Geometry check sheet. Reference: the model listing, model coordinates, mm. A direction names the side the tool comes from. Round coordinates to 2 decimals unless told otherwise and drop trailing zeros. Loops run counter-clockwise (first coordinate to the right, second up) from the corner with the lowest first, then second, coordinate; pieces in that order, holes last. Notation, with made-up numbers: (52.5, 42) - (80.5, 42) arc R31 cw to (80.5, 75) - close; hole circle Ø6 at (40.5, 63). An arc over 180 degrees is marked (long way). Answer as CSV lines item,"result". Start each with the question number.
1) Cross-section at B-B on x = 0. Record the boundary of the cut face in (y, z).
2) Depth check by flat-ended pin: P1, Ø1, axis at x = 1.5, z = 2.5, coming from the +Y side; P2, Ø4, axis at x = 4, y = 6.5, coming from the +Z side; P3, Ø3.5, axis at x = 0, z = 0, coming from the +Y side; P4, Ø2, axis at y = 20, z = 1.5, coming from the +X side. Enter the tip coordinate at first touch or a pass-through.
3) Cross-section at A-A on z = 0. Record the boundary of the cut face in (x, y).
4) Cross-section at C-C on y = 7. Record the boundary of the cut face in (x, z).
5) Draft check along Z on faces 3 (the flat face through (-2.1, 0, 4.3)), 4 (the cylindrical face through (0.9, 17.6, 2.86)), 5 (the cylindrical face through (-9.76, 12.32, -2.17)). Enter one of: released by +Z, released by -Z, zero draft, split by the parting line, or undercut.
6) Cross-section at D-D on y = 15.5. Record the boundary of the cut face in (x, z), and give its area (3 significant figures).
7) Thickness scan on line 1 along X through (y, z) = (7.25, 0); line 2 along X through (y, z) = (14, 0); line 3 along Y through (x, z) = (-4, 2). Record the ranges inside material, lowest first.
8) Access from +Z, -Z, +X, -X, +Y, -Y to the whole of each face (thin tool, end or side, straight path). Record for faces 1 (the flat face through (2.4, 25, 2.1)), 2 (the cylindrical face through (1.352, 4.93, -4.292)).
from build123d import *

# Parameters (mm, degrees)
SKETCH1_R           = 10
BOSS_EXTRUDE1_DEPTH = 25
SKETCH3_R           = 3
CUT_EXTRUDE1_DEPTH  = 29.722813233
SKETCH4_R           = 4.5
CUT_EXTRUDE2_DEPTH  = 10


with BuildPart() as part:
    # Sketch1 → Boss-Extrude1 (new body)
    with BuildSketch(Plane(origin=(0, 0, 0), x_dir=(1, 0, 0), z_dir=(0, 1, 0))):
        with Locations(Location((0, 0, 0), (0, 0, 270))):
            Circle(SKETCH1_R)
    extrude(amount=BOSS_EXTRUDE1_DEPTH)

    # Sketch3 → Cut-Extrude1 (cut, through all)
    with BuildSketch(Plane(origin=(0, 25, 0), x_dir=(1, 0, 0), z_dir=(0, 1, 0))):
        with Locations(Location((0, 0, 0), (0, 0, 270))):
            Circle(SKETCH3_R)
    extrude(amount=-CUT_EXTRUDE1_DEPTH, mode=Mode.SUBTRACT)

    # Sketch4 → Cut-Extrude2 (cut)
    with BuildSketch(Plane.XZ):
        with Locations(Location((0, 0, 0), (0, 0, 270))):
            Circle(SKETCH4_R)
    extrude(amount=-CUT_EXTRUDE2_DEPTH, mode=Mode.SUBTRACT)


solid = part.part
Answer block:
1,outline,"(0, -10) - (25, -10) - (25, -3) - (10, -3) - (10, -4.5) - (0, -4.5) - close; (0, 4.5) - (10, 4.5) - (10, 3) - (25, 3) - (25, 10) - (0, 10) - close"
2,P1,"stops at y = 25"
2,P2,"stops at z = 9.8"
2,P3,"passes through"
2,P4,"stops at x = 9.99"
3,outline,"(-10, 0) - (-4.5, 0) - (-4.5, 10) - (-3, 10) - (-3, 25) - (-10, 25) - close; (3, 10) - (4.5, 10) - (4.5, 0) - (10, 0) - (10, 25) - (3, 25) - close"
4,outline,"circle Ø20 at (0, 0); hole circle Ø9 at (0, 0)"
5,face 3,"zero draft"
5,face 4,"undercut"
5,face 5,"split by the parting line"
6,outline,"circle Ø20 at (0, 0); hole circle Ø6 at (0, 0)"
6,area,"286 mm^2"
7,line 1,"x = -10 to -4.5, 4.5 to 10"
7,line 2,"x = -10 to -3, 3 to 10"
7,line 3,"y = 10 to 25"
8,face 1,"+Z, -Z, +X, -X, +Y"
8,face 2,"-Y"
